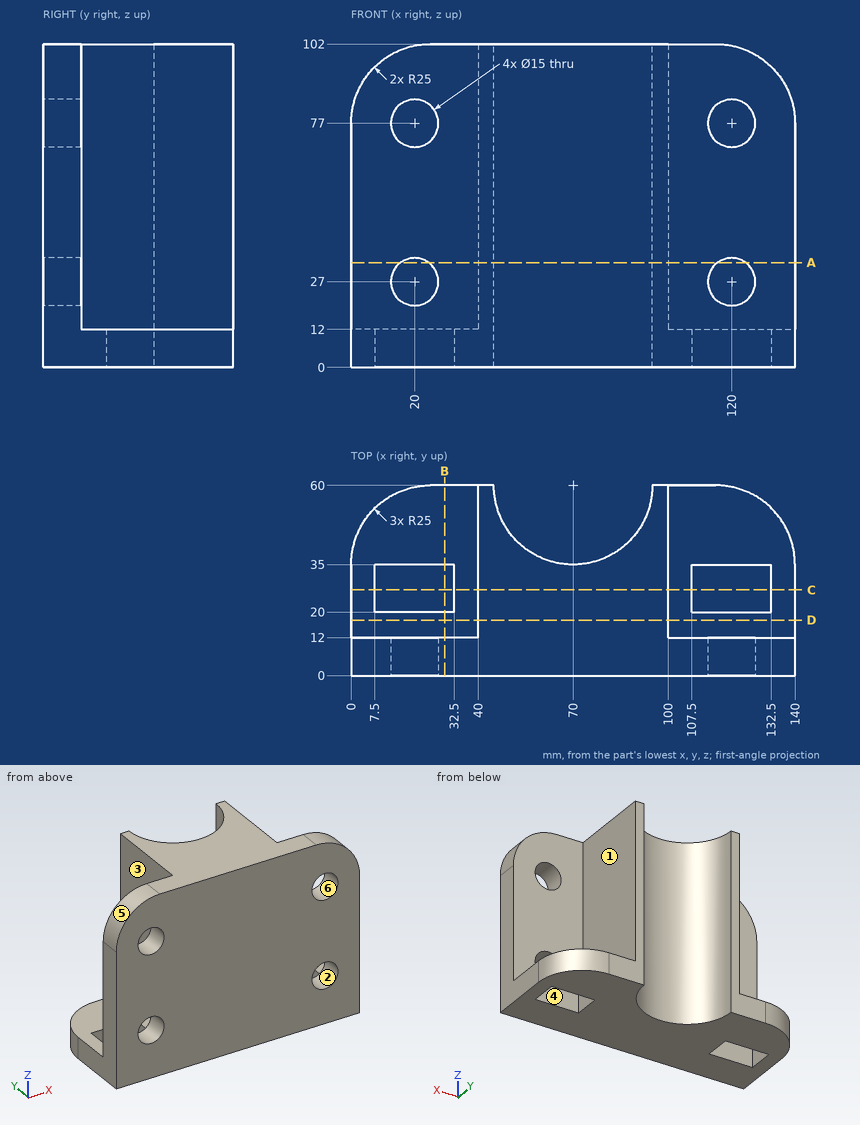
Answer from the drawing. Dimensions are ordinates in mm from the lowest x, y and z of the part. A direction names the side the tool comes from. Round coordinates to 2 decimals unless told otherwise and drop trailing zeros. Write each loop counter-clockwise with the first axis right and the second up, starting at its lowest first coordinate (ties: lowest second). Pieces come first, ordered by that corner, then holes. Notation, with made-up numbers: M 54.5,29 L 112.5,29 A24 ccw 112.5,47 Z; hole C 8,-6.5 d11. An arc over 180 degrees is marked long. Write each question's results on one line, items separated by ' | '. Start each with the question number.
Item 1: Find section A-A on z = 33. Write down the section's boundary in (x, y).
Item 2: Straight lines are drawn through the part: probe 1 along X at (y, z) = (4.5, 77); probe 2 along Z at (x, y) = (20, 8); probe 3 along X at (y, z) = (12.5, 79). For each, find the intervals that lie inside material, in ascending order.
Item 3: Which of the six approach directions +Z, -Z, +X, -X, +Y, -Y give full straight-line access (tool end or side, diameter ignored) to the marked faces 1, 2 and 3?
Item 4: Given pin 1 Ø9.5 at (x, z) = (22, 7.5) entering from +Y; pin 2 Ø8 at (y, z) = (31, 57.5) entering from +X; pin 3 Ø12 at (x, z) = (27.5, 48.5) entering from +Y; pin 4 Ø1.5 at (x, y) = (22.5, 7.5) entering from +Z, each flat-ended and moving along its own axis, determine where each tip first touches the part or whether it passes through.
Item 5: Find section D-D on y = 17.5. Write down the section's boundary in (x, z), and give its area (3 significant figures).
Item 6: Find section B-B on x = 29.5. Write down the section's boundary in (y, z).
Item 7: The mould has two halves that part along Z. Classify the marked faces 4, 5 and 6: +Z half, -Z half, draft (parallel to the pull), parting line (faces both ways), or undercut.
Item 8: Find section C-C on y = 27. Write down the section's boundary in (x, z), and give its area (3 significant figures).
Answer block:
1) outline: M 0,0 L 15.5,0 L 15.5,12 L 0,12 Z; M 24.5,0 L 115.5,0 L 115.5,12 L 100,12 L 100,60 L 95,60 A25 cw 45,60 L 40,60 L 40,12 L 24.5,12 Z; M 124.5,0 L 140,0 L 140,12 L 124.5,12 Z
2) probe 1: x = 0 to 12.5, 27.5 to 112.5, 127.5 to 140 | probe 2: z = 0 to 19.5, 34.5 to 69.5, 84.5 to 101.49 | probe 3: x = 40 to 100
3) face 1: +Z, +X, +Y | face 2: +Y, -Y | face 3: +Z, -X, +Y
4) pin 1: stops at y = 60 | pin 2: stops at x = 100 | pin 3: stops at y = 12 | pin 4: stops at z = 101.94
5) outline: M 0,0 L 140,0 L 140,12 L 100,12 L 100,102 L 40,102 L 40,12 L 0,12 Z | area: 7,080 mm²
6) outline: M 0,0 L 20,0 L 20,12 L 12,12 L 12,102 L 0,102 Z; M 35,0 L 60,0 L 60,12 L 35,12 Z
7) face 4: draft | face 5: +Z half | face 6: undercut
8) outline: M 0,0 L 7.5,0 L 7.5,12 L 0,12 Z; M 32.5,0 L 107.5,0 L 107.5,12 L 100,12 L 100,102 L 40,102 L 40,12 L 32.5,12 Z; M 132.5,0 L 140,0 L 140,12 L 132.5,12 Z | area: 6,480 mm²
